```python
from build123d import *

# Parameters (mm, degrees)
F0_W          = 406.4
F0_H          = 558.8
F1_DEPTH      = 76.2
F3_DEPTH      = 406.4
F4_R          = 38.09999
F5_W          = 393.7
F5_H          = 374.65
F6_DEPTH      = 19.05
F8_DEPTH      = 406.4
F8_DEPTH_BACK = 6.35
F9_W          = 393.7
F9_H          = 146.05
F10_DEPTH     = 25.4
F12_DEPTH     = 6.35
F14_DEPTH     = 6.35
F15_R         = 3.175
F16_DEPTH     = 406.401
F17_R         = 5.08
F18_W         = 6.35
F18_H         = 38.1
F19_DEPTH     = 381


# Not quite as in the source:
# - a fillet or chamfer is up to 0.001 mm smaller than in the source, because OpenCascade refuses the exact size


with BuildPart() as f1:
    # F0 (on Top) → F1 (new body)
    with BuildSketch(Plane.XY):
        with Locations((-259.8249833828, -5.0296476896)):
            Rectangle(F0_W, F0_H)
    extrude(amount=F1_DEPTH)

    # F2 (on face) → F3 (cut)
    with BuildSketch(Plane(origin=(-463.0249833828, 0, 0), x_dir=(0, -1, 0), z_dir=(-1, 0, 0))):
        Polygon((5.0296476896, 76.2), (-147.3703523104, 76.2), (-96.5703523104, 38.1), (5.0296476896, 38.1), align=None)
        Polygon((157.4296476896, 76.2), (5.0296476896, 76.2), (5.0296476896, 38.1), (106.6296476896, 38.1), align=None)
        Polygon((-147.3703523104, 76.2), (-274.3703523104, 76.2), (-274.3703523104, 38.1), (-96.5703523104, 38.1), align=None)
    extrude(amount=-F3_DEPTH, mode=Mode.SUBTRACT)

    # F4 (radius 38.1 in the source; OpenCascade refuses exactly that, so slightly less here)
    f4_edges = [f1.edges().sort_by_distance(p)[0] for p in [
        (-56.624983, -5.029648, 0),
        (-463.024983, -5.029648, 0),
    ]]
    fillet(f4_edges, radius=F4_R)

    # F5 (on face) → F6 (cut)
    with BuildSketch(Plane.XY.offset(38.1)):
        with Locations((-259.8249833828, 80.6953523104)):
            Rectangle(F5_W, F5_H)
    extrude(amount=-F6_DEPTH, mode=Mode.SUBTRACT)

    # F7 (on face) → F8 (cut, two sides)
    with BuildSketch(Plane.YZ.offset(-56.6249833828)) as f8_sk:
        Polygon((-278.0796476896, 76.2), (-278.0796476896, 44.45), (-125.6796476896, 44.45), (-168.012981023, 76.2), align=None)
    extrude(amount=-F8_DEPTH, mode=Mode.SUBTRACT)
    extrude(f8_sk.sketch, amount=F8_DEPTH_BACK, mode=Mode.SUBTRACT)

    # F9 (on face) → F10 (cut)
    with BuildSketch(Plane.XY.offset(44.45)):
        with Locations((-259.8249833828, -205.0546476896)):
            Rectangle(F9_W, F9_H)
    extrude(amount=-F10_DEPTH, mode=Mode.SUBTRACT)

    # F11 (on face) → F12 (join)
    with BuildSketch(Plane.YZ.offset(-56.6249833828)):
        Polygon((-168.012981023, 76.2), (-278.0796476896, 76.2), (-278.0796476896, 44.45), (-125.6796476896, 44.45), align=None)
    extrude(amount=-F12_DEPTH)

    # F13 (on face) → F14 (join)
    with BuildSketch(Plane(origin=(-463.0249833828, 0, 0), x_dir=(0, -1, 0), z_dir=(-1, 0, 0))):
        Polygon((168.012981023, 76.2), (125.6796476896, 44.45), (278.0796476896, 44.45), (278.0796476896, 76.2), align=None)
    extrude(amount=-F14_DEPTH)

    # F15 (on face) → F16 (cut, through all)
    with BuildSketch(Plane.YZ.offset(-56.6249833828)):
        with Locations((-220.9296476896, 57.15)):
            Circle(F15_R)
    extrude(amount=-F16_DEPTH, mode=Mode.SUBTRACT)

    # F17
    f17_edges = [f1.edges().sort_by_distance(p)[0] for p in [
        (-463.024983, -220.929648, 76.2),
        (-259.824983, -157.429648, 76.2),
        (-259.824983, -284.429648, 76.2),
        (-56.624983, -220.929648, 76.2),
    ]]
    fillet(f17_edges, radius=F17_R)

    # F18 (on face) → F19 (join, through all)
    with BuildSketch(Plane(origin=(0, 274.3703523104, 0), x_dir=(-1, 0, 0), z_dir=(0, 1, 0))):
        with Locations((259.8249833828, 19.05)):
            Rectangle(F18_W, F18_H)
    extrude(amount=-F19_DEPTH)


solid = f1.part
```
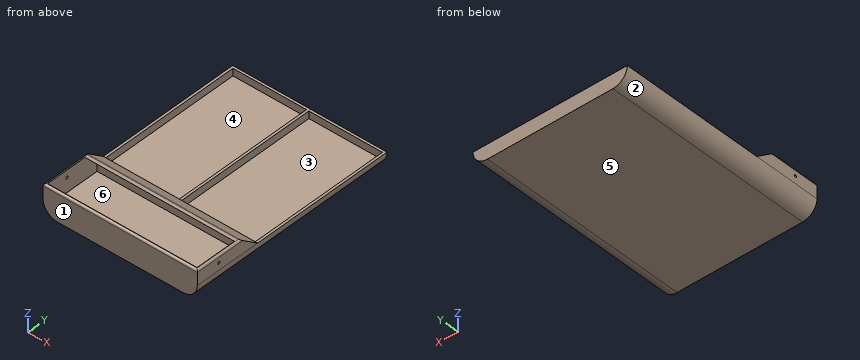
Geometry check sheet. Reference: the model listing, model coordinates, mm. Face numbers are marked on the shaded views. A direction names the side the tool comes from. Coordinates: 2 decimals unless noted, no trailing zeros. Order: outer loops, then holes, each group sorted by start corner. A loop starts at its lowest first (then second) coordinate and runs counter-clockwise, first axis right, second up.
Q1. Sectioned sample at A-A on x = -287.5. Record the cut outline in (y, z).
Reply:
outline: (-284.43, 0) - (274.37, 0) - (274.37, 38.1) - (268.02, 38.1) - (268.02, 19.05) - (-106.63, 19.05) - (-106.63, 38.1) - (-156.07, 75.18) arc R5.08 ccw to (-159.12, 76.2) - (-168.01, 76.2) - (-125.68, 44.45) - (-132.03, 44.45) - (-132.03, 19.05) - (-278.08, 19.05) - (-278.08, 76.2) - (-279.35, 76.2) arc R5.08 ccw to (-284.43, 71.12) - close
Q2. Draft check along X on the marked faces 1, 2 and 3. Enter one of: released by +X, released by -X, zero draft, split by the parting line, or undercut.
Reply:
face 1: zero draft
face 2: released by -X
face 3: undercut
Q3. Thickness scan on probe 1 along X at (y, z) = (-242, 49.5); probe 2 along X at (y, z) = (164, 20); probe 3 along Z at (x, y) = (-350, 175). Record the ranges inside material, lowest first.
Reply:
probe 1: x = -463.02 to -456.67, -62.97 to -56.62
probe 2: x = -458.45 to -456.67, -263 to -256.65, -62.97 to -61.2
probe 3: z = 0 to 19.05
Q4. Depth check by flat-ended pin: pin 1 Ø9.5 at (y, z) = (133.5, 27) entering from -X; pin 2 Ø2 at (y, z) = (-151, 22.5) entering from -X; pin 3 Ø1.5 at (x, z) = (-303.5, 57.5) entering from +Y. Enter the tip coordinate at first touch or a pass-through.
Reply:
pin 1: stops at x = -462.49
pin 2: stops at x = -460.12
pin 3: stops at y = -131.5
Q5. Tool access check on the marked faces 4, 5 and 6. Record the directions out of +Z, -Z, +X, -X, +Y, -Y that give a thin tool (end or side, any length) a straight path to the whole face; none if there is none.
Reply:
face 4: +Z
face 5: -Z, +X, -X, +Y, -Y
face 6: none
